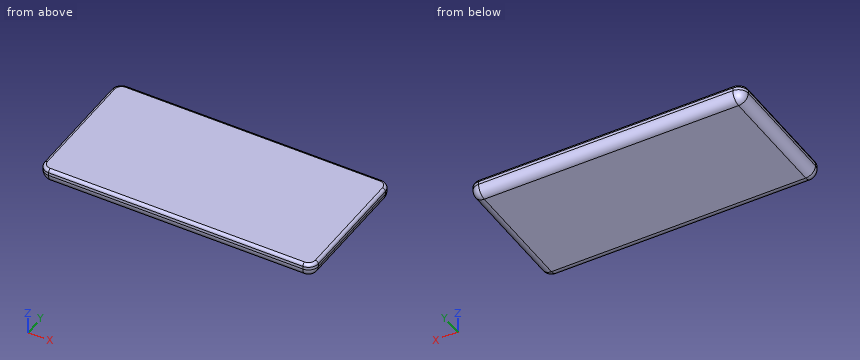
from build123d import *

# Parameters (mm, degrees)
F1_DEPTH = 8
F2_R     = 1.5
F3_R     = 5


with BuildPart() as f1:
    # F0 (on Top) → F1 (new body)
    with BuildSketch(Plane.XY):
        with BuildLine():
            Line((65.2941119671, 34.5224887133), (-65.2941119671, 34.5224887133))
            ThreePointArc((-65.2941119671, 34.5224887133), (-68.829645873, 33.0580226192), (-70.2941119671, 29.5224887133))
            Line((-70.2941119671, 29.5224887133), (-70.2941119671, -29.5224887133))
            ThreePointArc((-70.2941119671, -29.5224887133), (-68.829645873, -33.0580226192), (-65.2941119671, -34.5224887133))
            Line((-65.2941119671, -34.5224887133), (65.2941119671, -34.5224887133))
            ThreePointArc((65.2941119671, -34.5224887133), (68.829645873, -33.0580226192), (70.2941119671, -29.5224887133))
            Line((70.2941119671, -29.5224887133), (70.2941119671, 29.5224887133))
            ThreePointArc((70.2941119671, 29.5224887133), (68.829645873, 33.0580226192), (65.2941119671, 34.5224887133))
        make_face()
    extrude(amount=F1_DEPTH)

    # F2
    f2_edges = [f1.edges().sort_by_distance(p)[0] for p in [
        (0, 34.522489, 8),
        (-68.829646, 33.058023, 8),
        (-70.294112, 0, 8),
        (-68.829646, -33.058023, 8),
        (0, -34.522489, 8),
        (68.829646, -33.058023, 8),
        (70.294112, 0, 8),
        (68.829646, 33.058023, 8),
    ]]
    fillet(f2_edges, radius=F2_R)

    # F3
    f3_edges = [f1.edges().sort_by_distance(p)[0] for p in [
        (0, 34.522489, 0),
        (-68.829646, 33.058023, 0),
        (-70.294112, 0, 0),
        (-68.829646, -33.058023, 0),
        (0, -34.522489, 0),
        (68.829646, -33.058023, 0),
        (70.294112, 0, 0),
        (68.829646, 33.058023, 0),
    ]]
    fillet(f3_edges, radius=F3_R)


solid = f1.part
The listing builds one solid part. Answer for the finished solid, in the listing's coordinates (mm). Round coordinates to 2 decimals unless told otherwise and drop trailing zeros. Order: outer loops, then holes, each group sorted by start corner. A loop starts at its lowest first (then second) coordinate and runs counter-clockwise, first axis right, second up. Notation, with made-up numbers: M 41,15.25 L 96,15.25 A21 cw 96,32.25 Z; hole C -39,86.25 d11. An arc over 180 degrees is marked long. Answer in a Markdown table with one row per item. Add a question column.
1) Consider line 1 along Y through (x, z) = (-56, 4.5); line 2 along X through (y, z) = (5, 4.5); line 3 along Y through (x, z) = (-41.5, 3.5). Determine where each line is inside the solid, lowest interval first. Write a range as from..to.
2) The part is cut by section A-A on x = 4.5. Determine the outline of the cut face in (y, z).
3) Flat-ended cylindrical pins translate along their axes: pin 1 Ø1.5 at (y, z) = (22, 2.5) entering from +X; pin 2 Ø3 at (y, z) = (-8.5, 3) entering from -X; pin 3 Ø1 at (x, z) = (-16, 1) entering from -Y. Find the tip coordinate at first contact, or state that the pin passes through.
4) The part is cut by section B-B on z = 2. Determine the outline of the cut face in (x, y), plus the area to 3 significant figures.
Findings below:
| question | item | result |
|---|---|---|
| 1 | line 1 | y = -34.5..34.5 |
| 1 | line 2 | x = -70.27..70.27 |
| 1 | line 3 | y = -34.29..34.29 |
| 2 | outline | M -34.52,5 A5 ccw -29.52,0 L 29.52,0 A5 ccw 34.52,5 L 34.52,6.5 A1.5 ccw 33.02,8 L -33.02,8 A1.5 ccw -34.52,6.5 Z |
| 3 | pin 1 | stops at x = 69.98 |
| 3 | pin 2 | stops at x = -70.27 |
| 3 | pin 3 | stops at y = -33.09 |
| 4 | outline | M -69.29,-29.52 A4 ccw -65.29,-33.52 L 65.29,-33.52 A4 ccw 69.29,-29.52 L 69.29,29.52 A4 ccw 65.29,33.52 L -65.29,33.52 A4 ccw -69.29,29.52 Z |
| 4 | area | 9,280 mm² |
